For this review, take the finished solid that the model builds, in its own axes (mm). A direction names the side the tool comes from. Coordinates: 2 decimals unless noted, no trailing zeros. Order: outer loops, then holes, each group sorted by start corner. A loop starts at its lowest first (then second) coordinate and runs counter-clockwise, first axis right, second up. Notation, with made-up numbers: (10, 73.25) - (67, 73.25) arc R23 cw to (67, 96.25) - close; hole circle Ø10 at (4.5, 17.5). An arc over 180 degrees is marked (long way). One line per item, written item: value. Start each with the question number.
(1) To check wall thickness, follow line 1 along Z through (x, y) = (0, 3.75); line 2 along Y through (x, z) = (-28.5, -11.5); line 3 along Z through (x, y) = (14.5, 4). State the ranges of each line that lie inside material, in increasing order.
(2) Consider section C-C on z = 17. Write out the cut boundary in (x, y).
(3) Consider section A-A on z = 0. Write out the cut boundary in (x, y), then the cut area to 3 significant figures.
(4) Consider section D-D on x = -31. Write out the cut boundary in (y, z).
(5) Consider section B-B on x = 0. Write out the cut boundary in (y, z).
(6) For faces 1 (the flat face through (22.4, -3, 0.5)), 2 (the cylindrical face through (35.3, 1.6, 0)), 3 (the flat face through (3, 3.4, -27)), 4 (the cylindrical face through (-4.791, -0.535, -21.574)), 5 (the cylindrical face through (28.27, -0.27, -1.22)), list the 3-axis set-ups (+Z, -Z, +X, -X, +Y, -Y) from which the entire face can be reached by the end or side of a thin tool; tool diameter is ignored.
(7) Mouldability with a two-part tool opening along X and no side actions: class faces 6 (the cylindrical face through (-32.2, 0.2, -0.9)), 7 (the flat face through (-27, 0, 22)), 8 (the cylindrical face through (32.716, -1.479, 10.303)) as released by +X, released by -X, zero draft, split by the parting line, or undercut.
(8) Clearance check with flat-ended pins moving along their axes: pin 1 (4 mm diameter, centred on y = 2.5, z = 6, fed in from -X); pin 2 (6 mm diameter, centred on x = -19.5, y = 1.5, fed in from +Z); pin 3 (13.5 mm diameter, centred on x = 8, z = -7, fed in from -Y); pin 4 (4 mm diameter, centred on x = 5, z = 28.5, fed in from +Y). State where each tip first meets the part, or that it passes through.
```python
from build123d import *

# Parameters (mm, degrees)
F0_R      = 34.3
F1_DEPTH  = 3
F2_R      = 36.2
F3_DEPTH  = 3.4
F4_R      = 26.7
F5_DEPTH  = 4.8
F6_R      = 20
F7_DEPTH  = 6.2
F8_R      = 22.1
F9_DEPTH  = 5
F10_R     = 1.5
F11_DEPTH = 6.4
F13_R     = 1.6
F14_DEPTH = 1.9
F15_R     = 1.25
F16_DEPTH = 15


with BuildPart() as f1:
    # F0 (on Front) → F1 (new body)
    with BuildSketch(Plane.XZ):
        Circle(F0_R)
    extrude(amount=F1_DEPTH)

    # F2 (on face) → F3 (join)
    with BuildSketch(Plane(origin=(0, 0, 0), x_dir=(-1, 0, 0), z_dir=(0, 1, 0))):
        Circle(F2_R)
    extrude(amount=F3_DEPTH)

    # F4 (on face) → F5 (join)
    with BuildSketch(Plane(origin=(0, 3.4, 0), x_dir=(-1, 0, 0), z_dir=(0, 1, 0))):
        Circle(F4_R)
    extrude(amount=F5_DEPTH)

    # F6 (on face) → F7 (cut)
    with BuildSketch(Plane(origin=(0, 8.2, 0), x_dir=(-1, 0, 0), z_dir=(0, 1, 0))):
        Circle(F6_R)
    extrude(amount=-F7_DEPTH, mode=Mode.SUBTRACT)

    # F8 (on face) → F9 (cut)
    with BuildSketch(Plane.XZ.offset(3)):
        Circle(F8_R)
    extrude(amount=-F9_DEPTH, mode=Mode.SUBTRACT)

    # F10 (on face) → F11 (cut)
    with BuildSketch(Plane.XZ.offset(3)):
        with Locations((-31, 0)):
            Circle(F10_R)
    extrude(amount=-F11_DEPTH, mode=Mode.SUBTRACT)

    # F13 (on offset) → F14 (cut)
    with BuildSketch(Plane.YZ.offset(36.2)):
        Circle(F13_R)
    extrude(amount=-F14_DEPTH, mode=Mode.SUBTRACT)

    # F15 (on offset) → F16 (cut)
    with BuildSketch(Plane.YZ.offset(36.2)):
        Circle(F15_R)
    extrude(amount=-F16_DEPTH, mode=Mode.SUBTRACT)


solid = f1.part
```
Geometry check:
1. line 1: z = -26.7 to -20, 20 to 26.7
1. line 2: y = -3 to 3.4
1. line 3: z = -22.42 to -13.77, 13.77 to 22.42
2. outline: (-31.96, 0) - (-29.79, 0) - (-29.79, -3) - (-14.12, -3) - (-14.12, 2) - (-10.54, 2) - (-10.54, 8.2) - (-20.59, 8.2) - (-20.59, 3.4) - (-31.96, 3.4) - close; (10.54, 2) - (14.12, 2) - (14.12, -3) - (29.79, -3) - (29.79, 0) - (31.96, 0) - (31.96, 3.4) - (20.59, 3.4) - (20.59, 8.2) - (10.54, 8.2) - close
3. outline: (-36.2, 0) - (-34.3, 0) - (-34.3, -3) - (-32.5, -3) - (-32.5, 3.4) - (-36.2, 3.4) - close; (-29.5, -3) - (-22.1, -3) - (-22.1, 2) - (-20, 2) - (-20, 8.2) - (-26.7, 8.2) - (-26.7, 3.4) - (-29.5, 3.4) - close; (20, 2) - (22.1, 2) - (22.1, 1.25) - (34.3, 1.25) - (34.3, 1.6) - (36.2, 1.6) - (36.2, 3.4) - (26.7, 3.4) - (26.7, 8.2) - (20, 8.2) - close; (22.1, -3) - (34.3, -3) - (34.3, -1.25) - (22.1, -1.25) - close
3. area: 187 mm^2
4. outline: (-3, -14.68) - (0, -14.68) - (0, -18.69) - (3.4, -18.69) - (3.4, -1.5) - (-3, -1.5) - close; (-3, 1.5) - (3.4, 1.5) - (3.4, 18.69) - (0, 18.69) - (0, 14.68) - (-3, 14.68) - close
5. outline: (-3, -34.3) - (0, -34.3) - (0, -36.2) - (3.4, -36.2) - (3.4, -26.7) - (8.2, -26.7) - (8.2, -20) - (2, -20) - (2, -22.1) - (-3, -22.1) - close; (-3, 22.1) - (2, 22.1) - (2, 20) - (8.2, 20) - (8.2, 26.7) - (3.4, 26.7) - (3.4, 36.2) - (0, 36.2) - (0, 34.3) - (-3, 34.3) - close
6. face 1: +Z, -Z, +X, -X, -Y
6. face 2: +X, -Y
6. face 3: +Y
6. face 4: -Y
6. face 5: +X
7. face 6: undercut
7. face 7: zero draft
7. face 8: split by the parting line
8. pin 1: stops at x = -35.98
8. pin 2: stops at z = 32.22
8. pin 3: passes through
8. pin 4: stops at y = 3.4
